Verification items for the finished model (mm, model axes). Face numbers are marked on the shaded views. Coordinates: 2 decimals unless noted, no trailing zeros. Order: outer loops, then holes, each group sorted by start corner. A loop starts at its lowest first (then second) coordinate and runs counter-clockwise, first axis right, second up. Notation, with made-up numbers: M 74.5,10 L 101.5,10 A29 ccw 101.5,31 Z; hole C -40,29.5 d7. An arc over 180 degrees is marked long. Return JSON: item names as keys, results as strings.
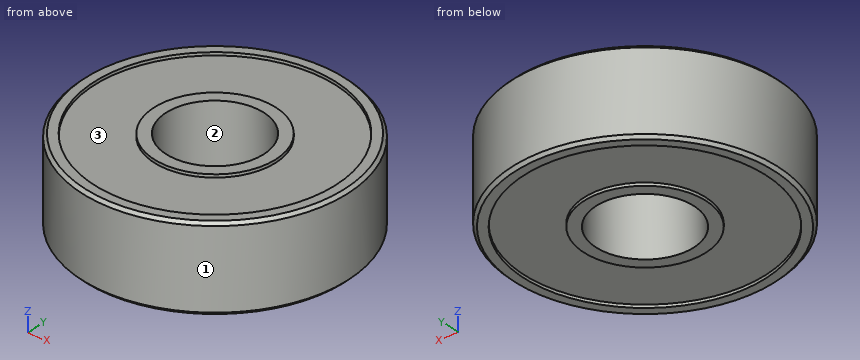
Autodesk Inventor part; units mm, degrees
ref_plane "YZ Plane" through (0, 0, 0) normal (1, 0, 0) x (0, 1, 0)
ref_plane "XZ Plane" through (0, 0, 0) normal (0, 1, 0) x (-1, 0, 0)
ref_plane "XY Plane" through (0, 0, 0) normal (0, 0, 1) x (1, 0, 0)
sketch "Sketch1" plane through (0, 0, 0) normal (0, 0, 1) x (1, 0, 0)
  circle A0 centre (0, 0) radius 11.025
  circle A1 centre (0, 0) radius 4.05
  dimension "d0" = 22.05
  dimension "d1" = 8.1
extrude "Extrusion1" add sketch "Sketch1" along normal blind 7
sketch "Sketch2" plane through (0, 0, 7) normal (0, 0, 1) x (1, 0, 0)
  circle A0 centre (0, 0) radius 5.05
  circle A1 centre (0, 0) radius 10.025
  circle A2 centre (0, 0) radius 11.025
  circle A3 centre (0, 0) radius 4.05
  dimension "d4" = 1
  dimension "d5" = 1
extrude "Extrusion2" cut sketch "Sketch2" against normal blind 0.25 contours A1
sketch "Sketch3" plane through (0, 0, 0) normal (0, 0, -1) x (-1, 0, 0)
  circle A0 centre (0, 0) radius 10.025
  circle A1 centre (0, 0) radius 5.05
extrude "Extrusion3" cut sketch "Sketch3" against normal blind 0.25
chamfer "Chamfer1" distance 0.25 angle 45 2 edges at (-11.025, 0, 7) (-11.025, 0, 0)
properties part number "bearing_22x8x7"
Q1. Go/stop test with flat-tipped pins: pin 1 (3 mm diameter, centred on x = 7.5, z = 2.5, fed in from +Y); pin 2 (3 mm diameter, centred on x = -8.5, z = 5, fed in from +Y). Record where each tip stops, or that it passes through.
Values:
{"pin 1": "y = 9.25", "pin 2": "y = 8.52"}
Q2. Cross-section at C-C, the plane z = 5.5. Record the boundary of the cut face in (x, y) (3 decimals).
Values:
{"outline": "C 0,0 d22.05; hole C 0,0 d8.1"}
Q3. Material ranges on line 1 along Y through (x, z) = (0, 0.1) (3 decimals); line 2 along Y through (x, z) = (0, 6.8) (3 decimals); line 3 along Y through (x, z) = (0, 2.75) (3 decimals), recorded low to high.
Values:
{"line 1": "-10.875 to -10.025, -5.05 to -4.05, 4.05 to 5.05, 10.025 to 10.875", "line 2": "-10.975 to -10.025, -5.05 to -4.05, 4.05 to 5.05, 10.025 to 10.975", "line 3": "-11.025 to -4.05, 4.05 to 11.025"}
Q4. Cross-section at A-A, the plane y = 0. Record the boundary of the cut face in (x, z) (3 decimals), and give its area (4 significant figures).
Values:
{"outline": "M -11.025,0.25 L -10.775,0 L -10.025,0 L -10.025,0.25 L -5.05,0.25 L -5.05,0 L -4.05,0 L -4.05,7 L -5.05,7 L -5.05,6.75 L -10.025,6.75 L -10.025,7 L -10.775,7 L -11.025,6.75 Z; M 4.05,0 L 5.05,0 L 5.05,0.25 L 10.025,0.25 L 10.025,0 L 10.775,0 L 11.025,0.25 L 11.025,6.75 L 10.775,7 L 10.025,7 L 10.025,6.75 L 5.05,6.75 L 5.05,7 L 4.05,7 Z", "area": "92.55 mm^2"}
Q5. Draft check along X on the marked faces 1, 2 and 3. Enter one of: pulls with the +X half, pulls with the -X half, needs draft (parallel to the pull), parting line crosses it, or undercut.
Values:
{"face 1": "parting line crosses it", "face 2": "undercut", "face 3": "undercut"}
